```python
from build123d import *

# Parameters (mm, degrees)
F1_DEPTH  = 100
F2_R      = 25
F3_DEPTH  = 30
F4_R      = 25
F5_DEPTH  = 30
F7_DEPTH  = 30
F10_W     = 20
F10_H     = 20
F11_DEPTH = 20


with BuildPart() as f1:
    # F0 (on Front) → F1 (new body)
    with BuildSketch(Plane.XZ):
        Polygon((-150, -50), (150, -50), (175, 50), (150, 50), (-150, 50), (-175, 50), align=None)
    extrude(amount=-F1_DEPTH)

    # F2 (on face) → F3 (cut)
    with BuildSketch(Plane.XZ):
        with Locations((50, 0)):
            Circle(F2_R)
        with Locations((-50, 0)):
            Circle(F2_R)
    extrude(amount=-F3_DEPTH, mode=Mode.SUBTRACT)

    # F4 (on face) → F5 (cut)
    with BuildSketch(Plane(origin=(0, 0, -50), x_dir=(1, 0, 0), z_dir=(0, 0, -1))):
        with Locations((0, -50)):
            Circle(F4_R)
    extrude(amount=-F5_DEPTH, mode=Mode.SUBTRACT)

    # F6 (on face) → F7 (cut)
    with BuildSketch(Plane.XY.offset(50)):
        Polygon((30, 100), (0, 100), (-30, 100), (-30, 70), (30, 70), align=None)
    extrude(amount=-F7_DEPTH, mode=Mode.SUBTRACT)

    # F10 (on face) → F11 (join)
    with BuildSketch(Plane(origin=(0, 0, -50), x_dir=(1, 0, 0), z_dir=(0, 0, -1))):
        with Locations((140, -10)):
            Rectangle(F10_W, F10_H)
        with Locations((140, -90)):
            Rectangle(F10_W, F10_H)
        with Locations((-140, -90)):
            Rectangle(F10_W, F10_H)
        with Locations((-140, -10)):
            Rectangle(F10_W, F10_H)
    extrude(amount=F11_DEPTH)


solid = f1.part
```
Geometry check sheet. Reference: the model listing, model coordinates, mm. A direction names the side the tool comes from. Coordinates: 2 decimals unless noted, no trailing zeros. Write each loop counter-clockwise with the first axis right and the second up, starting at its lowest first coordinate (ties: lowest second). Pieces come first, ordered by that corner, then holes. Notation, with made-up numbers: M -14,-7.5 L -1,-7.5 A5 ccw -1,0.5 Z; hole C 42,64.25 d5. An arc over 180 degrees is marked long. One line per item, written item: value. Start each with the question number.
(1) Sectioned sample at B-B, the plane y = 16. Enter the section's corners in (x, z), and give its area (3 significant figures).
(2) Sectioned sample at D-D, the plane y = 43. Enter the section's corners in (x, z).
(3) Tool access check on faces 5 (the face through (130, 90, -60)), 6 (the face through (-50, 30, 0)), 7 (the face through (-150, 90, -60)). Record the directions out of +Z, -Z, +X, -X, +Y, -Y that give a thin tool (end or side, any length) a straight path to the whole face; none if there is none.
(4) Sectioned sample at A-A, the plane z = -63. Enter the section's corners in (x, y), and give its area (3 significant figures).
(5) Depth check by flat-ended pin: pin 1 (4 mm diameter, centred on x = -125.5, y = 84, fed in from -Z); pin 2 (4 mm diameter, centred on y = 45, z = 0.5, fed in from -X) (3 decimals); pin 3 (6 mm diameter, centred on y = 10.5, z = -61, fed in from -X). Enter the tip coordinate at first touch or a pass-through.
(6) Release check for a two-part mould opening along X. For faces 1 (the face through (0, 50, -20)), 2 (the face through (140, 20, -60)), 3 (the face through (162.325, 49.3, -0.7)), 4 (the face through (30, 85, 35)) record: released by +X, released by -X, zero draft, split by the parting line, or undercut.
(7) Scan lines: line 1 along Y through (x, z) = (0, -43); line 2 along Z through (x, y) = (50, 18.25); line 3 along X through (y, z) = (14, 10). Record each from-to range of solid material in increasing order. Write a range as [from, to].
(8) Sectioned sample at C-C, the plane x = 0. Enter the section's corners in (y, z), and give its area (3 significant figures).
Filled sheet:
1. outline: M -175,50 L -150,-50 L -150,-70 L -130,-70 L -130,-50 L 130,-50 L 130,-70 L 150,-70 L 150,-50 L 175,50 Z; hole C -50,0 d50; hole C 50,0 d50
1. area: 29,400 mm²
2. outline: M -175,50 L -150,-50 L -24,-50 L -24,-20 L 24,-20 L 24,-50 L 150,-50 L 175,50 Z
3. face 5: -Z, +Y, -Y
3. face 6: -Y
3. face 7: -Z, -X, +Y, -Y
4. outline: M -150,0 L -130,0 L -130,20 L -150,20 Z; M -150,80 L -130,80 L -130,100 L -150,100 Z; M 130,0 L 150,0 L 150,20 L 130,20 Z; M 130,80 L 150,80 L 150,100 L 130,100 Z
4. area: 1,600 mm²
5. pin 1: z = -50
5. pin 2: x = -163.125
5. pin 3: x = -150
6. face 1: undercut
6. face 2: zero draft
6. face 3: released by +X
6. face 4: undercut
7. line 1: [0, 25], [75, 100]
7. line 2: [-50, -25], [25, 50]
7. line 3: [-165, -72.91], [-27.09, 27.09], [72.91, 165]
8. outline: M 0,-50 L 25,-50 L 25,-20 L 75,-20 L 75,-50 L 100,-50 L 100,20 L 70,20 L 70,50 L 0,50 Z
8. area: 7,600 mm²
